from build123d import *

# Parameters (mm, degrees)
F3_DEPTH        = 20
F3_COPIES_COUNT = 6


# Not quite as in the source:
# - a pattern or mirror of a feature is missing from the dataset's text; its kind, count and spacing are read off the source's solid


with BuildPart() as f1:
    # F0 (on Front) → F1 (revolve)
    with BuildSketch(Plane.XZ):
        Polygon((-13.5, -3), (-10.5, -3), (-10.5, 17), (-13.5, 17), (-13.5, 3), (-16.5, 3), (-16.5, 0), (-13.5, 0), align=None)
    revolve(axis=Axis((0, 0, 29.5368466722), (0, 0, 1)))

    # F2 (on face) → F3 (join, through all)
    with BuildSketch(Plane.XY.offset(17)):
        with BuildLine():
            ThreePointArc((0.3999274311, 10.4923809524), (0, 10.5), (-0.3999274311, 10.4923809524))
            ThreePointArc((-0.3999274311, 10.4923809524), (0, 10.1), (0.3999274311, 10.4923809524))
        make_face()
    f3 = extrude(amount=-F3_DEPTH)

    # F3_copies: F3 ×6 about axis
    f3_copies_axis = Axis((0, 0, 0), (0, 0, 1))
    for i in range(1, F3_COPIES_COUNT):
        add(f3.rotate(f3_copies_axis, i * 360 / F3_COPIES_COUNT))


solid = f1.part
Model file for the job. Use its own axes, mm. A direction names the side the tool comes from. Give positions to 0.01 mm unless a question says otherwise; leave off trailing zeros. Loops run counter-clockwise (first coordinate to the right, second up) from the corner with the lowest first, then second, coordinate; pieces in that order, holes last. Notation, with made-up numbers: (-2, 75) -> (48, 75) arc R10 cw to (48, 90) -> close; hole circle Ø7 at (20.5, 45). An arc over 180 degrees is marked (long way). Use a Markdown table: item, result. Add a question column.
(1) Slice it at B-B on y = 0. List the corners of the cut face in (x, z).
(2) Wall check: line 1 along Y through (x, z) = (-0.5, -0.5); line 2 along X through (y, z) = (0, 4.25); line 3 along Z through (x, y) = (9.5, 12.5). Give the ranges that are in metal, low to high.
(3) Mould opens along Y. For faces 6 (the cylindrical face through (2.93, 13.18, -1.52)), 7 (the cylindrical face through (-10.5, 0.1, 7.1)), 8 (the flat face through (-14, 0, 3)) say: +Y half, -Y half, draft (parallel to the pull), parting line (faces both ways), or undercut.
(4) Slice it at A-A on x = 4. List the corners of the cut face in (y, z).
(5) Drop flat-ended pins along their axis: pin 1 Ø12 at (y, z) = (-10, 10.5) entering from +X; pin 2 Ø1 at (y, z) = (5.5, 7.5) entering from -X; pin 3 Ø3 at (y, z) = (-9, 9) entering from -X (3 decimals). Give the stop position or say it passes through.
(6) Slice it at D-D on x = 12.5. List the corners of the cut face in (y, z), and give its area (3 significant figures).
(7) Tool access for faces 1 (the flat face through (14, 0, 0)), 2 (the cylindrical face through (10.5, -0.1, 7.1)), 3 (the cylindrical face through (2.93, 13.18, 9.9)), 4 (the flat face through (8.9, -5.1, 17)), 5 (the flat face through (-8.9, -5.1, -3)): list every direction of +Z, -Z, +X, -X, +Y, -Y with a clear straight run to the whole face (end or side of a thin tool).
(8) Slice it at C-C on z = 12. List the corners of the cut face in (x, y), and give its area (3 significant figures).
Filled sheet:
| question | item | result |
|---|---|---|
| 1 | outline | (-16.5, 0) -> (-13.5, 0) -> (-13.5, -3) -> (-10.5, -3) -> (-10.5, 17) -> (-13.5, 17) -> (-13.5, 3) -> (-16.5, 3) -> close; (10.5, -3) -> (13.5, -3) -> (13.5, 0) -> (16.5, 0) -> (16.5, 3) -> (13.5, 3) -> (13.5, 17) -> (10.5, 17) -> close |
| 2 | line 1 | -13.49 to -10.49, 10.49 to 13.49 |
| 2 | line 2 | -13.5 to -10.5, 10.5 to 13.5 |
| 2 | line 3 | 0 to 3 |
| 3 | face 6 | parting line |
| 3 | face 7 | undercut |
| 3 | face 8 | draft |
| 4 | outline | (-16.01, 0) -> (-12.89, 0) -> (-12.89, -3) -> (-9.71, -3) -> (-9.71, 17) -> (-12.89, 17) -> (-12.89, 3) -> (-16.01, 3) -> close; (9.71, -3) -> (12.89, -3) -> (12.89, 0) -> (16.01, 0) -> (16.01, 3) -> (12.89, 3) -> (12.89, 17) -> (9.71, 17) -> close |
| 5 | pin 1 | x = 12.89 |
| 5 | pin 2 | x = -12.54 |
| 5 | pin 3 | x = -11.225 |
| 6 | outline | (-10.77, 0) -> (-5.1, 0) -> (-5.1, -3) -> (5.1, -3) -> (5.1, 0) -> (10.77, 0) -> (10.77, 3) -> (5.1, 3) -> (5.1, 17) -> (-5.1, 17) -> (-5.1, 3) -> (-10.77, 3) -> close |
| 6 | area | 238 mm2 |
| 7 | face 1 | -Z |
| 7 | face 2 | +Z, -Z |
| 7 | face 3 | +Z |
| 7 | face 4 | +Z, +X, -X, +Y, -Y |
| 7 | face 5 | -Z, +X, -X, +Y, -Y |
| 8 | outline | circle Ø27 at (0, 0); hole (-9.29, -4.9) arc R0.4 cw to (-8.89, -5.59) arc R10.5 ccw to (-0.4, -10.49) arc R0.4 cw to (0.4, -10.49) arc R10.5 ccw to (8.89, -5.59) arc R0.4 cw to (9.29, -4.9) arc R10.5 ccw to (9.29, 4.9) arc R0.4 cw to (8.89, 5.59) arc R10.5 ccw to (0.4, 10.49) arc R0.4 cw to (-0.4, 10.49) arc R10.5 ccw to (-8.89, 5.59) arc R0.4 cw to (-9.29, 4.9) arc R10.5 ccw to start |
| 8 | area | 228 mm2 |
